```python
from build123d import *

# Parameters (mm, degrees)
SKETCH_1_R      = 2.5
SKETCH_1_R_2    = 3.4
EXTRUDE_1_DEPTH = 1000


with BuildPart() as part:
    # 草图1 → 凸台-拉伸1 (new body)
    with BuildSketch(Plane.XY):
        with BuildLine():
            Line((-2.798233949, -17.227303989), (7.951766051, -17.227303989))
            ThreePointArc((7.951766051, -17.227303989), (8.658872832, -16.93441077), (8.951766051, -16.227303989))
            Line((8.951766051, -16.227303989), (8.951766051, -5.477303989))
            Line((8.951766051, -5.477303989), (6.651766051, -5.477303989))
            Line((6.651766051, -5.477303989), (6.651766051, -7.427303989))
            Line((6.651766051, -7.427303989), (0.851766051, -7.427303989))
            ThreePointArc((0.851766051, -7.427303989), (-1.748233949, -2.227303989), (0.851766051, 2.972696011))
            Line((0.851766051, 2.972696011), (6.651766051, 2.972696011))
            Line((6.651766051, 2.972696011), (6.651766051, 1.022696011))
            Line((6.651766051, 1.022696011), (8.951766051, 1.022696011))
            Line((8.951766051, 1.022696011), (8.951766051, 11.772696011))
            ThreePointArc((8.951766051, 11.772696011), (8.658872832, 12.479802792), (7.951766051, 12.772696011))
            Line((7.951766051, 12.772696011), (-2.798233949, 12.772696011))
            Line((-2.798233949, 12.772696011), (-2.798233949, 10.472696011))
            Line((-2.798233949, 10.472696011), (-0.848233949, 10.472696011))
            Line((-0.848233949, 10.472696011), (-0.848233949, 4.672696011))
            ThreePointArc((-0.848233949, 4.672696011), (-6.048233949, 2.072696011), (-11.248233949, 4.672696011))
            Line((-11.248233949, 4.672696011), (-11.248233949, 10.472696011))
            Line((-11.248233949, 10.472696011), (-9.298233949, 10.472696011))
            Line((-9.298233949, 10.472696011), (-9.298233949, 12.772696011))
            Line((-9.298233949, 12.772696011), (-20.048233949, 12.772696011))
            ThreePointArc((-20.048233949, 12.772696011), (-20.75534073, 12.479802792), (-21.048233949, 11.772696011))
            Line((-21.048233949, 11.772696011), (-21.048233949, 1.022696011))
            Line((-21.048233949, 1.022696011), (-18.748233949, 1.022696011))
            Line((-18.748233949, 1.022696011), (-18.748233949, 2.972696011))
            Line((-18.748233949, 2.972696011), (-12.948233949, 2.972696011))
            ThreePointArc((-12.948233949, 2.972696011), (-10.348233949, -2.227303989), (-12.948233949, -7.427303989))
            Line((-12.948233949, -7.427303989), (-18.748233949, -7.427303989))
            Line((-18.748233949, -7.427303989), (-18.748233949, -5.477303989))
            Line((-18.748233949, -5.477303989), (-21.048233949, -5.477303989))
            Line((-21.048233949, -5.477303989), (-21.048233949, -16.227303989))
            ThreePointArc((-21.048233949, -16.227303989), (-20.75534073, -16.93441077), (-20.048233949, -17.227303989))
            Line((-20.048233949, -17.227303989), (-9.298233949, -17.227303989))
            Line((-9.298233949, -17.227303989), (-9.298233949, -14.927303989))
            Line((-9.298233949, -14.927303989), (-11.248233949, -14.927303989))
            Line((-11.248233949, -14.927303989), (-11.248233949, -9.127303989))
            ThreePointArc((-11.248233949, -9.127303989), (-6.048233949, -6.527303989), (-0.848233949, -9.127303989))
            Line((-0.848233949, -9.127303989), (-0.848233949, -14.927303989))
            Line((-0.848233949, -14.927303989), (-2.798233949, -14.927303989))
            Line((-2.798233949, -14.927303989), (-2.798233949, -17.227303989))
        make_face()
        with Locations((-6.048233949, -2.227303989)):
            Circle(SKETCH_1_R, mode=Mode.SUBTRACT)
        with Locations((-16.148233949, -12.327303989)):
            Circle(SKETCH_1_R_2, mode=Mode.SUBTRACT)
        with Locations((4.051766051, -12.327303989)):
            Circle(SKETCH_1_R_2, mode=Mode.SUBTRACT)
        with Locations((4.051766051, 7.872696011)):
            Circle(SKETCH_1_R_2, mode=Mode.SUBTRACT)
        with Locations((-16.148233949, 7.872696011)):
            Circle(SKETCH_1_R_2, mode=Mode.SUBTRACT)
    extrude(amount=EXTRUDE_1_DEPTH)


solid = part.part
```
Work out the finished part from the listing and answer in its coordinate system (mm). Coordinates: 2 decimals unless noted, no trailing zeros.
1) A flat-ended cylindrical pin translates along its axis: pin 1 (0.7 mm diameter, centred on x = -20.5, z = 292, fed in from -Y). Find the tip coordinate at first contact, or state that the pin passes through.
Results:
pin 1: stops at y = -17.22
2) Section A-A (z = 714) is taken. Give the number of separate pieces and of enclosed holes in the cut face, plus the area to 3 significant figures.
Results:
separate pieces: 1
enclosed holes: 5
area: 358 mm2
3) Consider probe 1 along X at (y, z) = (-12, 61); probe 2 along Y at (x, z) = (-16, 817); probe 3 along X at (y, z) = (-8, 444). Determine where each line is inside the solid, lowest interval first.
Results:
probe 1: x = -21.05 to -19.53, -12.76 to -11.25, -0.85 to 0.67, 7.44 to 8.95
probe 2: y = -17.23 to -15.72, -8.93 to -7.43, 2.97 to 4.48, 11.27 to 12.77
probe 3: x = -21.05 to -10.17, -1.93 to 8.95
